Input: dimensioned drawing with shaded views. Units: mm. Origin: part minimum x, y, z. A direction names the side the tool comes from. Give positions to 0.01 mm unless a question says otherwise; leave off trailing zeros. Answer in a Markdown table with one row per item.
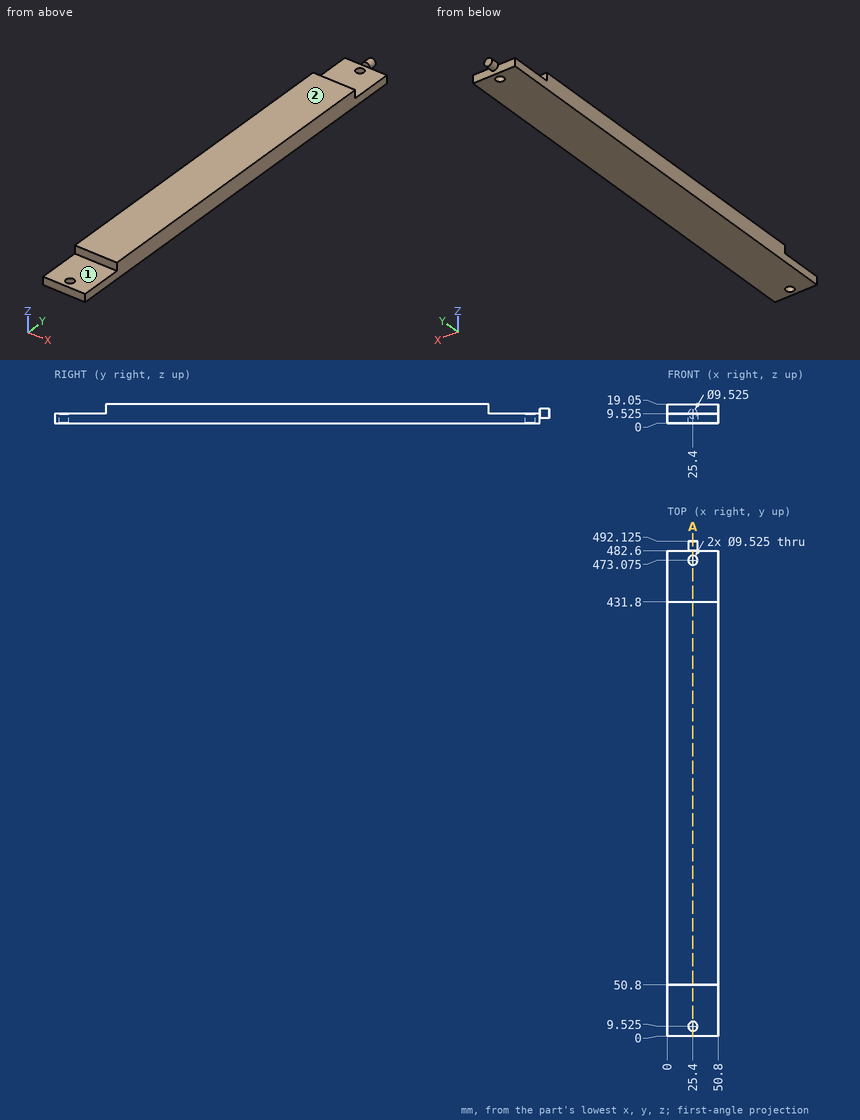
Q1. Section query A-A (x = 25.4). Give the number of separate pieces and of enclosed holes in the cut face, plus the area to 3 significant figures.
Values follow:
| item | result |
|---|---|
| separate pieces | 3 |
| enclosed holes | 0 |
| area | 8,140 mm^2 |
Q2. Reachability of the marked faces 1 and 2 from +Z, -Z, +X, -X, +Y, -Y: full face, straight path, thin tool, end or side. Return the list, or none.
Values follow:
| item | result |
|---|---|
| face 1 | +Z, +X, -X, -Y |
| face 2 | +Z, +X, -X, +Y, -Y |
Q3. Contact query for flat-ended pins moving along their axis: pin 1 Ø5 at (x, z) = (7, 8.5) entering from -Y; pin 2 Ø7.5 at (x, z) = (33, 3) entering from +Y; pin 3 Ø10 at (x, z) = (35.5, 15) entering from -Y; pin 4 Ø11 at (x, y) = (25.4, 473.075) entering from +Z (3 decimals). Output: stop coordinate, or through.
Values follow:
| item | result |
|---|---|
| pin 1 | y = 0 |
| pin 2 | y = 482.6 |
| pin 3 | y = 50.8 |
| pin 4 | z = 9.525 |
Q4. Ray query, probe 1 along Y at (x, z) = (25.4, 5.5) (1 decimal); probe 2 along Y at (x, z) = (25.4, 3.25); probe 3 along Y at (x, z) = (13, 10.75). Return the intervals inside material, ascending. Write a range as from..to.
Values follow:
| item | result |
|---|---|
| probe 1 | 0..4.8, 14.3..468.3, 477.8..492.1 |
| probe 2 | 0..4.76, 14.29..468.31, 477.84..482.6 |
| probe 3 | 50.8..431.8 |
